from build123d import *

# Parameters (mm, degrees)
ESQUISSE1_W             = 164
ESQUISSE1_H             = 215
BOSS_EXTRU_1_DEPTH      = 5
ESQUISSE2_W             = 25
ESQUISSE2_H             = 25
ENL_V_MAT_EXTRU_1_DEPTH = 5
CONG_1_R                = 5


with BuildPart() as part:
    # Esquisse1 → Boss.-Extru.1 (new body)
    with BuildSketch(Plane.XY):
        Rectangle(ESQUISSE1_W, ESQUISSE1_H)
    extrude(amount=BOSS_EXTRU_1_DEPTH)

    # Esquisse2 → Enlèv. mat.-Extru.1 (cut)
    with BuildSketch(Plane.XY):
        with Locations((-64.5, 90)):
            Rectangle(ESQUISSE2_W, ESQUISSE2_H)
        with Locations((64.5, 90)):
            Rectangle(ESQUISSE2_W, ESQUISSE2_H)
        with Locations((64.5, -90)):
            Rectangle(ESQUISSE2_W, ESQUISSE2_H)
        with Locations((-64.5, -90)):
            Rectangle(ESQUISSE2_W, ESQUISSE2_H)
    extrude(amount=ENL_V_MAT_EXTRU_1_DEPTH, mode=Mode.SUBTRACT)

    # Congé1
    cong_1_edges = [part.edges().sort_by_distance(p)[0] for p in [
        (-82, 107.5, 2.5),
        (82, 107.5, 2.5),
        (82, -107.5, 2.5),
        (-82, -107.5, 2.5),
    ]]
    fillet(cong_1_edges, radius=CONG_1_R)


solid = part.part
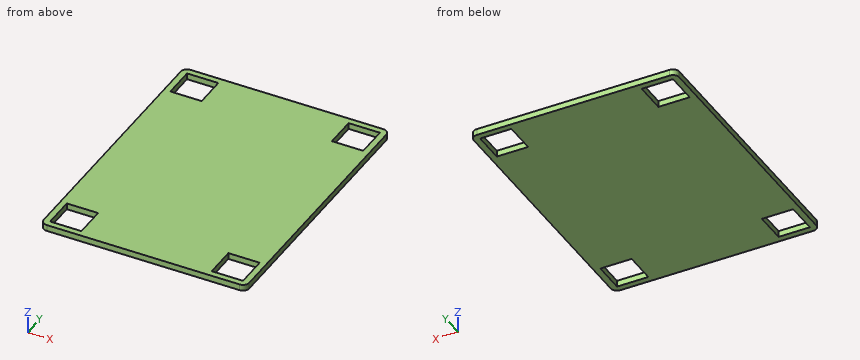
Work out the finished part from the listing and answer in its coordinate system (mm). Coordinates: 2 decimals unless noted, no trailing zeros. Write each loop counter-clockwise with the first axis right and the second up, starting at its lowest first coordinate (ties: lowest second). Pieces come first, ordered by that corner, then holes. Notation, with made-up numbers: M -15,8 L 8,8 A9 cw 8,23 Z; hole C 73.25,44.5 d1. An arc over 180 degrees is marked long. Answer as CSV lines item,"result". Start each with the question number.
Item 1: Section A-A on y = 90 is taken. Write down the section's boundary in (x, z), and give its area (3 significant figures).
Item 2: Consider L1, parallel to Y at x = -74.5, z = 1.2. Determine where the line is inside the solid, lowest interval first.
Item 3: Section C-C on x = 60.5 is taken. Write down the section's boundary in (y, z).
Item 4: Section B-B on z = 1.9 is taken. Write down the section's boundary in (x, y).
Checks:
1,outline,"M -82,0 L -77,0 L -77,5 L -82,5 Z; M -52,0 L 52,0 L 52,5 L -52,5 Z; M 77,0 L 82,0 L 82,5 L 77,5 Z"
1,area,"570 mm²"
2,L1,"y = -107.5 to -102.5, -77.5 to 77.5, 102.5 to 107.5"
3,outline,"M -107.5,0 L -102.5,0 L -102.5,5 L -107.5,5 Z; M -77.5,0 L 77.5,0 L 77.5,5 L -77.5,5 Z; M 102.5,0 L 107.5,0 L 107.5,5 L 102.5,5 Z"
4,outline,"M -82,-102.5 A5 ccw -77,-107.5 L 77,-107.5 A5 ccw 82,-102.5 L 82,102.5 A5 ccw 77,107.5 L -77,107.5 A5 ccw -82,102.5 Z; hole M -77,-102.5 L -52,-102.5 L -52,-77.5 L -77,-77.5 Z; hole M -77,77.5 L -52,77.5 L -52,102.5 L -77,102.5 Z; hole M 52,-102.5 L 77,-102.5 L 77,-77.5 L 52,-77.5 Z; hole M 52,77.5 L 77,77.5 L 77,102.5 L 52,102.5 Z"
